```python
from build123d import *

# Parameters (mm, degrees)
F1_DEPTH  = 38.1
F3_DEPTH  = 63.5
F4_R      = 3.175
F6_DEPTH  = 69.85
F6_FACE_R = 3.175
F7_DEPTH  = 18.542
F5_W      = 24.768822
F5_H      = 2.994034
F8_DEPTH  = 76.2
F8_FACE_W = 24.768822
F8_FACE_H = 2.994034
F9_DEPTH  = 53.34
F10_W     = 222.162876
F10_H     = 22.374636
F11_DEPTH = 50.8
F12_W     = 8.382
F12_H     = 3.175
F13_DEPTH = 69.85
F14_DEPTH = 50.546


with BuildPart() as f1:
    # F0 (on Front) → F1 (new body)
    with BuildSketch(Plane.XZ):
        with BuildLine():
            ThreePointArc((-32.499379, 0), (67.068651, 52.513153), (166.636681, 0))
            Line((166.636681, 0), (171.877104, 3.58615))
            ThreePointArc((171.877104, 3.58615), (67.068651, 58.863153), (-37.739801, 3.58615))
            Line((-37.739801, 3.58615), (-32.499379, 0))
        make_face()
    extrude(amount=-F1_DEPTH)

    # F2 (on Top) → F3 (cut)
    with BuildSketch(Plane.XY):
        with BuildLine():
            Line((105.508113, 24.880887), (31.848113, 24.880887))
            ThreePointArc((31.848113, 24.880887), (30.950088, 24.508913), (30.578113, 23.610887))
            Line((30.578113, 23.610887), (30.578113, 13.450887))
            ThreePointArc((30.578113, 13.450887), (30.950088, 12.552862), (31.848113, 12.180887))
            Line((31.848113, 12.180887), (105.508113, 12.180887))
            ThreePointArc((105.508113, 12.180887), (106.406139, 12.552862), (106.778113, 13.450887))
            Line((106.778113, 13.450887), (106.778113, 23.610887))
            ThreePointArc((106.778113, 23.610887), (106.406139, 24.508913), (105.508113, 24.880887))
        make_face()
    extrude(amount=F3_DEPTH, mode=Mode.SUBTRACT)

    # F4 (on Top) → F6 (join)
    with BuildSketch(Plane.XY):
        with Locations((-17.501814, 19.295603)):
            Circle(F4_R)
        with Locations((152.629465, 20.332575)):
            Circle(F4_R)
    extrude(amount=F6_DEPTH)

    # F6_face (on face) → F7 (cut)
    with BuildSketch(Plane(origin=(152.629465, 20.332575, 0), x_dir=(1, 0, 0), z_dir=(0, 0, -1))):
        Circle(F6_FACE_R)
        with Locations((-170.131279, 1.036972)):
            Circle(F6_FACE_R)
    extrude(amount=-F7_DEPTH, mode=Mode.SUBTRACT)

    # F5 (on Top) → F8 (join)
    with BuildSketch(Plane.XY):
        with Locations((69.149714, 32.560246)):
            Rectangle(F5_W, F5_H)
    extrude(amount=F8_DEPTH)

    # F8_face (on face) → F9 (cut)
    with BuildSketch(Plane(origin=(69.149714, 32.560246, 0), x_dir=(1, 0, 0), z_dir=(0, 0, -1))):
        Rectangle(F8_FACE_W, F8_FACE_H)
    extrude(amount=-F9_DEPTH, mode=Mode.SUBTRACT)

    # F10 (on Front) → F11 (cut)
    with BuildSketch(Plane.XZ):
        with Locations((66.641135, 7.16073)):
            Rectangle(F10_W, F10_H)
    extrude(amount=-F11_DEPTH, mode=Mode.SUBTRACT)

    # F12 (on Top) → F13 (join)
    with BuildSketch(Plane.XY):
        with Locations((44.929113, 7.840642)):
            Rectangle(F12_W, F12_H)
        with Locations((92.427113, 7.840642)):
            Rectangle(F12_W, F12_H)
    extrude(amount=F13_DEPTH)

    # F12 (on Top) → F14 (cut)
    with BuildSketch(Plane.XY):
        with Locations((44.929113, 7.840642)):
            Rectangle(F12_W, F12_H)
        with Locations((92.427113, 7.840642)):
            Rectangle(F12_W, F12_H)
    extrude(amount=F14_DEPTH, mode=Mode.SUBTRACT)


solid = f1.part
```
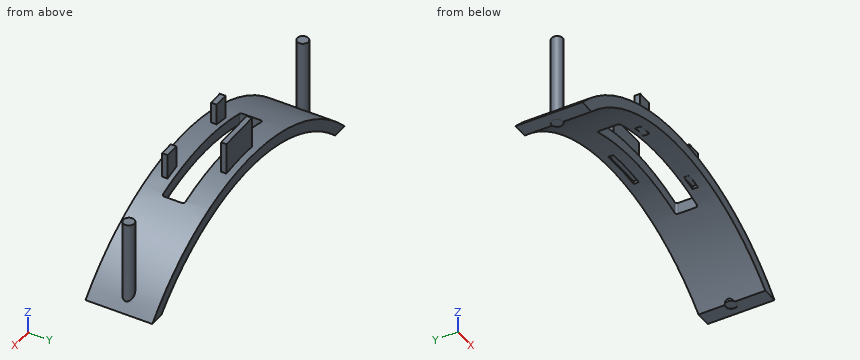
Read the model definition and answer for the solid it produces. Units are mm, in the model's axes. Coordinates: 2 decimals unless noted, no trailing zeros. Write each loop counter-clockwise with the first axis right and the second up, starting at its lowest first coordinate (ties: lowest second). Pieces come first, ordered by that corner, then holes. Notation, with made-up numbers: (-40, 48) - (18, 48) arc R13 ccw to (18, 61) - close; hole circle Ø6 at (-33, 30.5). An arc over 180 degrees is marked (long way). Answer as a JSON object with one key per item and string values. Group by question number.
1. Each of these flat-tipped pins is pushed along its axis until it touches: P1, Ø2, axis at y = 17.5, z = 51, coming from the -X side; P2, Ø1, axis at y = 17.5, z = 40, coming from the +X side; P3, Ø1, axis at y = 8, z = 64, coming from the -X side. Where does it stop, or does it pass through?
2. A cutting plane is placed at B-B (z = 42.5). Determine the outline of the cut face in (x, y) (3 decimals), plus the area to 3 significant figures.
3. A cutting plane is placed at C-C (y = 27). Determine the outline of the cut face in (x, z).
4. Consider L1, parallel to Y at x = 93, z = 50; L2, parallel to Z at x = 27.5, y = 31; L3, parallel to Y at x = 80, z = 60.5. Determine where each line is inside the solid, lowest interval first. Write a range as [from, to].
5. A cutting plane is placed at D-D (x = 119). Determine the outline of the cut face in (y, z), plus the area to 3 significant figures.
6. A cutting plane is placed at A-A (x = 34.5). Determine the outline of the cut face in (y, z).
Worked out:
{
 "1": {"P1": "stops at x = -20.58", "P2": "stops at x = 154.78", "P3": "stops at x = 40.74"},
 "2": {"outline": "circle Ø6.35 at (-17.502, 19.296); (4.711, 0) - (18.945, 0) - (18.945, 38.1) - (4.711, 38.1) - close; (115.193, 0) - (129.426, 0) - (129.426, 38.1) - (115.193, 38.1) - close; circle Ø6.35 at (152.629, 20.333)", "area": "1,150 mm²"},
 "3": {"outline": "(-25.93, 18.35) - (-17.05, 18.35) arc R120.65 cw to (151.19, 18.35) - (160.07, 18.35) arc R127 ccw to start"},
 "4": {"L1": "y = [0, 6.25], [9.43, 12.18], [24.88, 38.1]", "L2": "z = [45.84, 52.54]", "L3": "y = [31.06, 34.06]"},
 "5": {"outline": "(0, 40.76) - (38.1, 40.76) - (38.1, 47.76) - (0, 47.76) - close", "area": "267 mm²"},
 "6": {"outline": "(0, 48.03) - (12.18, 48.03) - (12.18, 54.62) - (0, 54.62) - close; (24.88, 48.03) - (38.1, 48.03) - (38.1, 54.62) - (24.88, 54.62) - close"}
}
